CAD build for the part. Positions are in the model's coordinates, mm. Round coordinates to 2 decimals unless told otherwise and drop trailing zeros. Order: outer loops, then holes, each group sorted by start corner. A loop starts at its lowest first (then second) coordinate and runs counter-clockwise, first axis right, second up. Notation, with made-up numbers: M 20,-31.5 L 55,-31.5 A33 ccw 55,5.5 Z; hole C 82,9.5 d1. An arc over 180 degrees is marked long. Put each result on its own line as item: value.
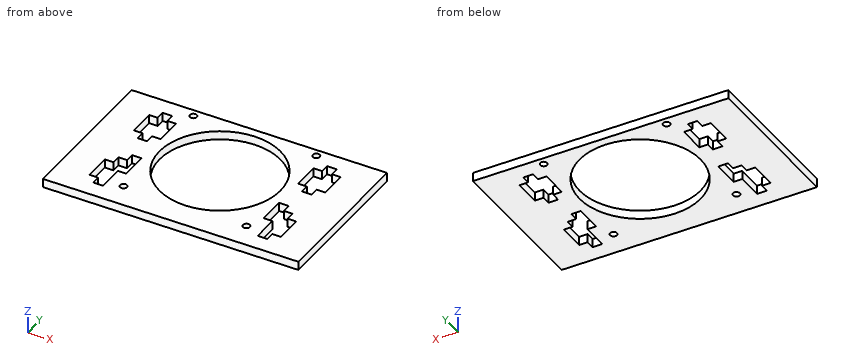
```python
from build123d import *

# Parameters (mm, degrees)
SKETCH2_R           = 35
SKETCH2_R_2         = 2
BOSS_EXTRUDE1_DEPTH = 5


with BuildPart() as part:
    # Sketch2 → Boss-Extrude1 (new body)
    with BuildSketch(Plane(origin=(0, 0, 0), x_dir=(-1, 0, 0), z_dir=(0, 0, -1))):
        Polygon((-144.276672243, 28.966950724), (-144.276672243, -46.033049276), (-144.276672243, -61.033049276), (3.323327757, -61.033049276), (3.323327757, -46.033049276), (3.323327757, 28.966950724), align=None)
        with Locations((-70.476672243, -11.033049276)):
            Circle(SKETCH2_R, mode=Mode.SUBTRACT)
        with Locations((-34.976672243, 24.466950724)):
            Circle(SKETCH2_R_2, mode=Mode.SUBTRACT)
        with Locations((-105.976672243, 24.466950724)):
            Circle(SKETCH2_R_2, mode=Mode.SUBTRACT)
        with Locations((-105.976672243, -46.533049276)):
            Circle(SKETCH2_R_2, mode=Mode.SUBTRACT)
        with Locations((-34.976672243, -46.533049276)):
            Circle(SKETCH2_R_2, mode=Mode.SUBTRACT)
        Polygon((-30.776672243, 14.266950724), (-25.776672243, 14.266950724), (-25.776672243, 19.266950724), (-20.176672243, 19.266950724), (-20.176672243, 14.266950724), (-15.176672243, 14.266950724), (-15.176672243, -1.333049276), (-20.176672243, -1.333049276), (-20.176672243, -6.333049276), (-25.776672243, -6.333049276), (-25.776672243, -1.333049276), (-30.776672243, -1.333049276), align=None, mode=Mode.SUBTRACT)
        Polygon((-115.176672243, -6.333049276), (-115.176672243, -1.333049276), (-110.176672243, -1.333049276), (-110.176672243, 14.266950724), (-115.176672243, 14.266950724), (-115.176672243, 19.266950724), (-120.776672243, 19.266950724), (-120.776672243, 14.266950724), (-125.776672243, 14.266950724), (-125.776672243, -1.333049276), (-120.776672243, -1.333049276), (-120.776672243, -6.333049276), align=None, mode=Mode.SUBTRACT)
        Polygon((-120.776672243, -25.733049276), (-115.776672243, -25.733049276), (-115.776672243, -20.733049276), (-110.176672243, -20.733049276), (-110.176672243, -36.333049276), (-115.176672243, -36.333049276), (-115.176672243, -51.333049276), (-120.776672243, -51.333049276), (-120.776672243, -46.333049276), (-125.776672243, -46.333049276), (-125.776672243, -30.733049276), (-120.776672243, -30.733049276), align=None, mode=Mode.SUBTRACT)
        Polygon((-25.776672243, -36.333049276), (-25.776672243, -51.333049276), (-20.176672243, -51.333049276), (-20.176672243, -46.333049276), (-15.176672243, -46.333049276), (-15.176672243, -30.733049276), (-20.176672243, -30.733049276), (-20.176672243, -25.733049276), (-25.176672243, -25.733049276), (-25.176672243, -20.733049276), (-30.776672243, -20.733049276), (-30.776672243, -36.333049276), align=None, mode=Mode.SUBTRACT)
    extrude(amount=BOSS_EXTRUDE1_DEPTH)


solid = part.part
```
Item 1: Pin check, flat tip, straight feed: P1, Ø2.5, axis at x = 105.98, y = -46.53, coming from the +Z side. Stop position of the tip, or through.
Answers below:
P1: through
Item 2: Probe line 1 along Y through (x, z) = (20, -0.9); line 2 along Y through (x, z) = (119, -2.2); line 3 along X through (y, z) = (-51, -1.2). List the from-to ranges inside material, lowest first. Write a range as [from, to].
Answers below:
line 1: [-61.03, -46.33], [-30.73, -1.33], [14.27, 28.97]
line 2: [-61.03, -51.33], [-25.73, -6.33], [19.27, 28.97]
line 3: [-3.32, 20.18], [25.78, 115.18], [120.78, 144.28]
Item 3: Band-saw the part on A-A on y = -38. Give the cut face in (x, z), and give its area (3 significant figures).
Answers below:
outline: M -3.32,-5 L 15.18,-5 L 15.18,0 L -3.32,0 Z; M 25.78,-5 L 48.17,-5 L 48.17,0 L 25.78,0 Z; M 92.79,-5 L 115.18,-5 L 115.18,0 L 92.79,0 Z; M 125.78,-5 L 144.28,-5 L 144.28,0 L 125.78,0 Z
area: 409 mm²
Item 4: Band-saw the part on C-C on x = 117.5. Give the cut face in (y, z), and give its area (3 significant figures).
Answers below:
outline: M -61.03,-5 L -51.33,-5 L -51.33,0 L -61.03,0 Z; M -25.73,-5 L -6.33,-5 L -6.33,0 L -25.73,0 Z; M 19.27,-5 L 28.97,-5 L 28.97,0 L 19.27,0 Z
area: 194 mm²
Item 5: Band-saw the part on B-B on x = 78.5. Give the cut face in (y, z).
Answers below:
outline: M -61.03,-5 L -45.1,-5 L -45.1,0 L -61.03,0 Z; M 23.03,-5 L 28.97,-5 L 28.97,0 L 23.03,0 Z
Item 6: Band-saw the part on D-D on y = -8. Give the cut face in (x, z) (3 decimals), and give its area (3 significant figures).
Answers below:
outline: M -3.323,-5 L 35.608,-5 L 35.608,0 L -3.323,0 Z; M 105.345,-5 L 144.277,-5 L 144.277,0 L 105.345,0 Z
area: 389 mm²
